Design review of the part built by this model. Coordinates are the model's own, in mm. A direction names the side the tool comes from. Round coordinates to 2 decimals unless told otherwise and drop trailing zeros. Order: outer loops, then holes, each group sorted by start corner. A loop starts at its lowest first (then second) coordinate and runs counter-clockwise, first axis right, second up. Notation, with made-up numbers: (59, 77.5) - (96, 77.5) arc R23 cw to (96, 108.5) - close; hole circle Ø6 at (-37.5, -32). An arc over 180 degrees is marked (long way). Write item = value, one per line.
from build123d import *

# Parameters (mm, degrees)
SKETCH_R              = 15
PAD_DEPTH             = 20
PAD001_DEPTH          = 45
POLARPATTERN_COUNT    = 3
CHAMFER_SIZE          = 3
CYLINDER_R            = 2.6
CYLINDER_DEPTH        = 30
POCKET_DEPTH          = 15
POLARPATTERN001_COUNT = 3


with BuildPart() as part:
    # Sketch → Pad (new body)
    with BuildSketch(Plane.XY):
        Circle(SKETCH_R)
    extrude(amount=PAD_DEPTH)

    # Sketch001 → Pad001 (join)
    with BuildSketch(Plane.YZ):
        with BuildLine():
            Line((-15, 0), (-7.5, 7.5))
            ThreePointArc((7.5, 7.5), (0, 10.606602), (-7.5, 7.5))
            Line((7.5, 7.5), (15, 0))
            Line((15, 0), (-15, 0))
        make_face()
    pad001 = extrude(amount=PAD001_DEPTH)

    # PolarPattern: Pad001 ×3 about axis
    polarpattern_axis = Axis((0, 0, 0), (0, 0, 1))
    for i in range(1, POLARPATTERN_COUNT):
        add(pad001.rotate(polarpattern_axis, i * 360 / POLARPATTERN_COUNT))

    # Chamfer
    chamfer_edges = [part.edges().sort_by_distance(p)[0] for p in [
        (-15, 0, 20),
    ]]
    chamfer(chamfer_edges, length=CHAMFER_SIZE)

    # Cylinder → Cylinder (cut)
    with BuildSketch(Plane.XY):
        Circle(CYLINDER_R)
    extrude(amount=CYLINDER_DEPTH, mode=Mode.SUBTRACT)

    # Sketch002 → Pocket (cut, symmetric)
    with BuildSketch(Plane.XZ):
        Polygon((15.5, 12), (47.5, 0), (47.5, 12), align=None)
    pocket = extrude(amount=POCKET_DEPTH, both=True, mode=Mode.SUBTRACT)

    # PolarPattern001: Pocket ×3 about axis
    polarpattern001_axis = Axis((0, 0, 0), (0, 0, 1))
    for i in range(1, POLARPATTERN001_COUNT):
        add(pocket.rotate(polarpattern001_axis, i * 360 / POLARPATTERN001_COUNT), mode=Mode.SUBTRACT)


solid = part.part
1) We need section D-D on z = 13.75. Write out the cut boundary in (x, y), and give its area (3 significant figures).
Findings:
outline = circle Ø30 at (0, 0); hole circle Ø5.2 at (0, 0)
area = 686 mm^2
2) We need section C-C on x = 22.5. Write out the cut boundary in (y, z) (3 decimals).
Findings:
outline = (-15, 0) - (15, 0) - (7.5, 7.5) arc R10.607 ccw to (4.961, 9.375) - (-4.961, 9.375) arc R10.607 ccw to (-7.5, 7.5) - close
3) To check wall thickness, follow L1, parallel to X at y = 0, z = 15; L2, parallel to Y at x = 0, z = 5.75. State the ranges of each line that lie inside material, in increasing order. Write a range as from..to.
Findings:
L1 = -15..-2.6, 2.6..15
L2 = -18.5..-2.6, 2.6..18.5
4) We need section A-A on x = -30.5. Write out the cut boundary in (y, z), and give its area (3 significant figures).
Findings:
outline = (-34.35, 0) - (-22.83, 0) - (-28.5, 2.84) - (-34.35, 0.94) - close; (22.83, 0) - (34.35, 0) - (34.35, 0.94) - (28.5, 2.84) - close
area = 38.2 mm^2
5) Clearance check with flat-ended pins moving along their axes: pin 1 Ø4 at (x, y) = (-17, 35.5) entering from +Z; pin 2 Ø1 at (y, z) = (19.5, 9) entering from +X; pin 3 Ø4 at (x, z) = (8.5, 5.5) entering from -Y. State where each tip first meets the part, or that it passes through.
Findings:
pin_1 = 3.85
pin_2 = -3.88
pin_3 = -13.52
6) The part is to be moulded in two halves that separate along Y. For faces 1 (the flat face through (-23.504, -16.438, 2.864)), 2 (the cylindrical face through (18.531, 0.117, 10.606)), 3 (the flat face through (-0.4, 24.97, 2.86)), say which applies: released by +Y, released by -Y, zero draft, split by the parting line, or undercut.
Findings:
face_1 = undercut
face_2 = split by the parting line
face_3 = released by +Y
7) For faces 4 (the flat face through (26, -12, 3)), 5 (the flat face through (-21.33, 12.88, 2.97)), 6 (the cylindrical face through (-3.252, -14.643, 11.065)), 7 (the flat face through (26, 12, 3)), list the 3-axis set-ups (+Z, -Z, +X, -X, +Y, -Y) from which the entire face can be reached by the end or side of a thin tool; tool diameter is ignored.
Findings:
face_4 = +Z, +X, -Y
face_5 = +Z, -X
face_6 = +Z
face_7 = +Z, +X, +Y
8) We need section B-B on z = 8.5. Write out the cut boundary in (x, y), and give its area (3 significant figures).
Findings:
outline = (-17.91, -18.33) - (-6.92, -24.68) - (-1.3, -14.94) arc R15 ccw to (13.59, -6.34) - (24.83, -6.34) - (24.83, 6.34) - (13.59, 6.34) arc R15 ccw to (-1.3, 14.94) - (-6.92, 24.68) - (-17.91, 18.33) - (-12.29, 8.6) arc R15 ccw to (-12.29, -8.6) - close; hole circle Ø5.2 at (0, 0)
area = 1,080 mm^2
